Build history of the part. All positions in model axes, mm. Round coordinates to 2 decimals unless told otherwise and drop trailing zeros. Loops run counter-clockwise (first coordinate to the right, second up) from the corner with the lowest first, then second, coordinate; pieces in that order, holes last. Notation, with made-up numbers: (65.25, 57) - (84.25, 57) arc R19 cw to (84.25, 64) - close; hole circle Ø9 at (58, 19.25). An arc over 180 degrees is marked (long way). Use a Markdown table: item, result.
Autodesk Inventor part; units mm, degrees
ref_plane "XZ Plane" through (0, 0, 0) normal (0, 1, 0) x (-1, 0, 0)
sketch "Sketch1" plane through (0, 0, 0) normal (0, 1, 0) x (-1, 0, 0)
  circle A0 centre (0, 0) radius 146.05
  circle A1 centre (0, 0) radius 184.15
  dimension "camInsideDiameter" = 292.1
  dimension "d1" = 368.3
extrude "Extrusion1" add sketch "Sketch1" along normal blind 12.7
sketch "Sketch2" plane through (0, 12.7, 0) normal (0, 1, 0) x (1, 0, 0)
  circle A0 centre (0, 0) radius 146.05 construction
  circle A1 centre (0, 0) radius 184.15 construction
  line L0 (0, 0) -> (147.2071, -39.444) construction
  line L1 (0, 0) -> (184.15, 0) construction
  line L2 (0, 0) -> (147.2071, 39.444) construction
  line L3 (147.2071, -39.444) -> (173.1094, -15.5967)
  line L4 (147.2071, 39.444) -> (173.1094, 15.5967)
  arc A2 (173.1094, -15.5967) -> (173.1094, 15.5967) centre (158.75, 0) ccw
  dimension "oneHalfPhase" = 15
  dimension "d5" = 15
  dimension "innerRadiusForCam" = 152.4
  dimension "innerRadisuForCam" = 152.4
  dimension "d12" = 158.75
sketch "Sketch8" plane through (0, 12.7, 0) normal (0, 1, 0) x (1, 0, 0)
  line L0 (0, 0) -> (184.15, 0) construction
  circle A0 centre (0, 0) radius 184.15 construction
  line L1 (0, 0) -> (177.8752, 47.6615) construction
  line L2 (0, 0) -> (47.6615, 177.8752) construction
  line L3 (0, 0) -> (0, 184.15) construction
  line L4 (0, 0) -> (177.8752, -47.6615) construction
  circle A1 centre (0, 0) radius 155.8689 construction
  circle A2 centre (0, 0) radius 173.9571 construction
  point P0 (150.5578, 40.3418)
  point P1 (168.0296, 45.0234)
  dimension "angleForCamMovement" = 15
  dimension "d17" = 15
  dimension "d18" = 15
sketch "Sketch9" plane through (0, 0, 0) normal (0, 0, 1) x (1, 0, 0)
  circle A0 centre (195.7327, 13.0626) radius 6.1855
  line L0 (-146.05, 12.7) -> (146.05, 12.7)
  point P0 (0, 0)
  dimension "d22" = 0.3625
ref_plane "Work Plane2" through (0, 12.7, 0) normal (-0.2588, 0, 0.9659) x (0.9659, 0, 0.2588)
ref_plane "Work Plane3" through (0, 12.7, 0) normal (0.2588, 0, 0.9659) x (0.9659, 0, -0.2588)
ref_plane "Work Plane4" through (0, 12.7, 0) normal (0.9659, 0, 0.2588) x (0.2588, 0, -0.9659)
sketch "Sketch11" plane through (0, 12.7, 0) normal (-0.2588, 0, 0.9659) x (0.9659, 0, 0.2588)
  circle A0 centre (163.1045, -0.0307) radius 7.9043
  point P0 (0, -12.7)
loft "Loft1" add profiles "Sketch11", "Sketch9"
sketch "Sketch7" plane through (0, 12.7, 0) normal (0, 1, 0) x (1, 0, 0)
  circle A0 centre (0, 0) radius 153.9875
  circle A1 centre (0, 0) radius 174.625
  line L0 (0, 0) -> (184.15, 0) construction
  circle A2 centre (0, 0) radius 184.15 construction
  line L1 (0, 0) -> (177.8752, 47.6615) construction
  arc A3 (174.625, 0) -> (148.7405, 39.8549) centre (134.2536, 2.1131) ccw
  arc A4 (148.7405, -39.8549) -> (174.625, 0) centre (134.2536, -2.1131) ccw
  dimension "d13" = 349.25
  dimension "d14" = 307.975
  dimension "d15" = 15
ref_plane "Work Plane1" through (147.2071, 12.7, 39.444) normal (0.7357, 0, -0.6773) x (0, 1, 0)
sketch "Sketch4" plane through (147.2071, 12.7, 39.444) normal (0.7357, 0, -0.6773) x (0, 1, 0)
  circle A0 centre (0, 0) radius 3.175
  point P0 (-12.7, -128.725)
  dimension "d9" = 6.35
sweep "Sweep1" cut profiles "Sketch4" path "Sketch2"
equation "\"d17\" = angleForCamMovement"
equation "\"d18\" = angleForCamMovement"
equation "\"d5\" = oneHalfPhase"
properties part number "DiskCam" material "PC/ABS Plastic"
Q1. Cut at B-B, the plane z = -53. List the corners of the cut face in (x, y), plus the area to 3 significant figures.
Results found:
| item | result |
|---|---|
| outline | (-176.36, 0) - (-136.09, 0) - (-136.09, 12.7) - (-176.36, 12.7) - close; (136.09, 0) - (176.36, 0) - (176.36, 12.7) - (136.09, 12.7) - close |
| area | 1,020 mm2 |
Q2. Drop flat-ended pins along their axis: pin 1 (3 mm diameter, centred on y = 4.5, z = -1.5, fed in from +X); pin 2 (10 mm diameter, centred on x = 163, y = 15.5, fed in from +Z); pin 3 (6 mm diameter, centred on x = -123.5, y = 11, fed in from +Z). Give the stop position or say it passes through.
Results found:
| item | result |
|---|---|
| pin 1 | stops at x = 184.15 |
| pin 2 | stops at z = 93.14 |
| pin 3 | stops at z = 139.25 |
Q3. Pull direction X, two halves, no side cores. Call faces 1 (the face through (-139.306, 6.261, -43.869)), 2 (the face through (196, 13, 0)): pulls with the +X half, pulls with the -X half, needs draft (parallel to the pull), parting line crosses it, or undercut.
Results found:
| item | result |
|---|---|
| face 1 | undercut |
| face 2 | needs draft |
Q4. Probe line 1 (Z direction, x = 0, y = 6.75); line 2 (Z direction, x = -57.5, y = 3.25); line 3 (Y direction, x = 0.5, z = -164.5). List the from-to ranges inside material, lowest first.
Results found:
| item | result |
|---|---|
| line 1 | z = -184.15 to -146.05, 146.05 to 184.15 |
| line 2 | z = -174.94 to -134.25, 134.25 to 174.94 |
| line 3 | y = 0 to 12.7 |
Q5. Cut at C-C, the plane z = 152.5. List the corners of the cut face in (x, y).
Results found:
| item | result |
|---|---|
| outline | (-103.22, 0) - (103.22, 0) - (103.22, 12.7) - (-103.22, 12.7) - close |
Q6. Cut at A-A, the plane x = 0. List the corners of the cut face in (y, z).
Results found:
| item | result |
|---|---|
| outline | (0, -184.15) - (12.7, -184.15) - (12.7, -146.05) - (0, -146.05) - close; (0, 146.05) - (12.7, 146.05) - (12.7, 184.15) - (0, 184.15) - close |
